Job drawing, mm, ordinate dimensions from the low corner. One solid piece. A direction names the side the tool comes from. Give positions to 0.01 mm unless a question says otherwise; leave off trailing zeros. Order: outer loops, then holes, each group sorted by start corner. A loop starts at its lowest first (then second) coordinate and runs counter-clockwise, first axis right, second up. Notation, with made-up numbers: M 81.25,-6.75 L 102.25,-6.75 A20 cw 102.25,12.25 Z; hole C 19.25,53 d1. An arc over 180 degrees is marked long. Put each result on its own line as item: value. Start each with the question number.
1) Cut at D-D (y = 26). Write the cut outline in (x, z).
2) Two-plate mould, pull along Y, no slides. Class the marked faces 1, 2 and 3: released by +Y, released by -Y, zero draft, split by the parting line, or undercut.
3) Drill centre lines: line 1 (X direction, y = 5, z = 2.6); line 2 (X direction, y = 20, z = 2.25); line 3 (Y direction, x = 11.25, z = 5) (1 decimal). Where is each one in solid material? Low to high. Write a range as [from, to].
4) Cut at B-B (x = 13). Write the cut outline in (y, z) (1 decimal), and give its area (3 significant figures).
5) Cut at A-A (z = 2.75). Give the number of separate pieces and of enclosed holes in the cut face.
6) Tool access for the marked faces 4, 5 and 6: list every direction of +Z, -Z, +X, -X, +Y, -Y with a clear straight run to the whole face (end or side of a thin tool).
7) Pin check, flat tips, straight feed: pin 1 (9.5 mm diameter, centred on x = 5, y = 5, fed in from +Z); pin 2 (2 mm diameter, centred on y = 24, z = 5, fed in from +X); pin 3 (2 mm diameter, centred on x = 9.5, z = 4, fed in from +Y); pin 4 (3 mm diameter, centred on x = 5.5, z = 1, fed in from +Y). Stop position of each tip, or through.
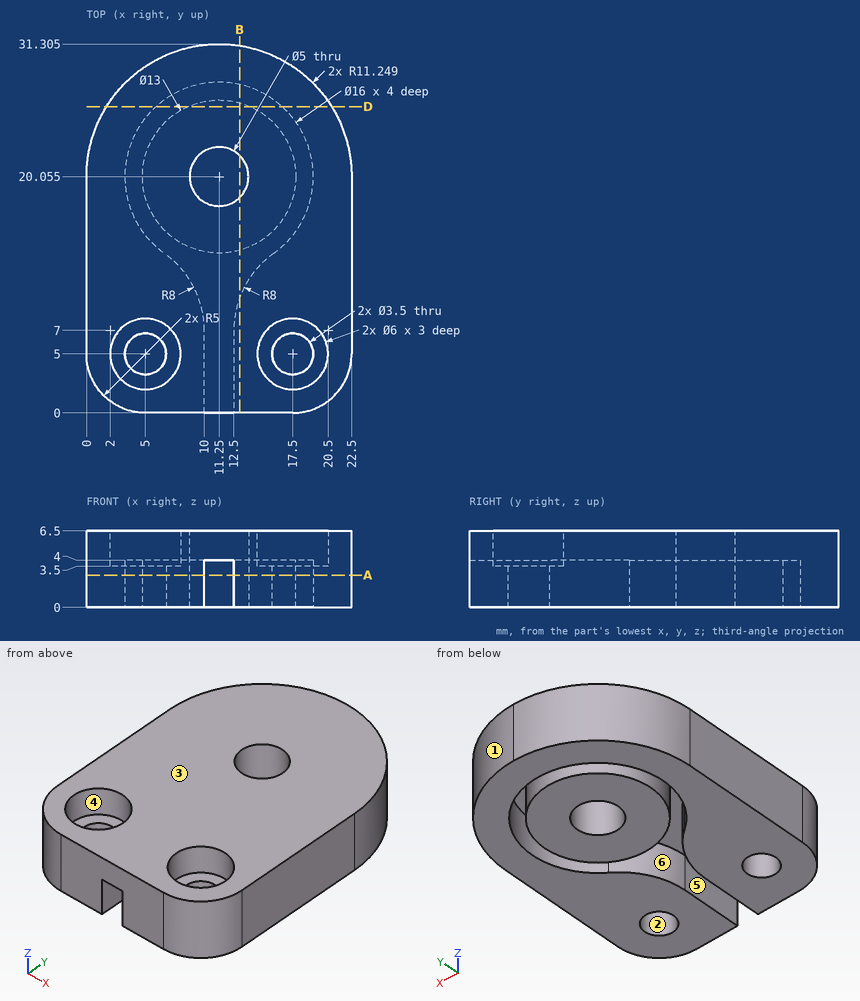
Solution:
1. outline: M 1.7,0 L 5.9,0 L 5.9,4 L 8.62,4 L 8.62,0 L 13.88,0 L 13.88,4 L 16.6,4 L 16.6,0 L 20.8,0 L 20.8,6.5 L 1.7,6.5 Z
2. face 1: released by +Y
2. face 2: undercut
2. face 3: zero draft
3. line 1: [0, 3.25], [6.75, 10], [12.5, 15.75], [19.25, 22.5]
3. line 2: [0, 3.25], [4.75, 8.75], [13.75, 17.75], [19.25, 22.5]
3. line 3: [0, 17.6], [22.6, 31.3]
4. outline: M 0,0 L 9.8,0 L 9.8,4 L 13.8,4 L 13.8,0 L 18.3,0 L 18.3,6.5 L 0,6.5 Z; M 21.8,0 L 26.3,0 L 26.3,4 L 27.9,4 L 27.9,0 L 31.2,0 L 31.2,6.5 L 21.8,6.5 Z
4. area: 157 mm²
5. separate pieces: 2
5. enclosed holes: 3
6. face 4: +Z
6. face 5: -Z, -Y
6. face 6: -Z
7. pin 1: z = 6.5
7. pin 2: x = 22.11
7. pin 3: y = 31.28
7. pin 4: y = 30.47
